```python
from build123d import *

# Parameters (mm, degrees)
SALIENTE_EXTRUIR1_DEPTH = 120
CROQUIS3_R              = 3.9
CORTAR_EXTRUIR1_DEPTH   = 32


with BuildPart() as part:
    # Croquis2 → Saliente-Extruir1 (new body)
    with BuildSketch(Plane(origin=(0, 0, 0), x_dir=(1, 0, 0), z_dir=(0, 1, 0))):
        with BuildLine():
            Line((-44.836996695, 15.45631068), (-20.836996695, 15.45631068))
            ThreePointArc((-20.836996695, 15.45631068), (-18.00856957, 14.284737804), (-16.836996695, 11.45631068))
            Line((-16.836996695, 11.45631068), (-16.836996695, -12.54368932))
            ThreePointArc((-16.836996695, -12.54368932), (-18.00856957, -15.372116445), (-20.836996695, -16.54368932))
            Line((-20.836996695, -16.54368932), (-44.836996695, -16.54368932))
            ThreePointArc((-44.836996695, -16.54368932), (-47.665423819, -15.372116445), (-48.836996695, -12.54368932))
            Line((-48.836996695, -12.54368932), (-48.836996695, 11.45631068))
            ThreePointArc((-48.836996695, 11.45631068), (-47.665423819, 14.284737804), (-44.836996695, 15.45631068))
        make_face()
    extrude(amount=SALIENTE_EXTRUIR1_DEPTH)

    # Croquis3 → Cortar-Extruir1 (cut)
    with BuildSketch(Plane.XY.offset(16.54368932)):
        with Locations((-32.836996695, 18)):
            Circle(CROQUIS3_R)
    extrude(amount=-CORTAR_EXTRUIR1_DEPTH, mode=Mode.SUBTRACT)


solid = part.part
```
The listing builds one solid part. Answer for the finished solid, in the listing's coordinates (mm). Give positions to 0.01 mm unless a question says otherwise; leave off trailing zeros. Order: outer loops, then holes, each group sorted by start corner. A loop starts at its lowest first (then second) coordinate and runs counter-clockwise, first axis right, second up.
1) Determine the mould class of faces 1 (the face through (-36.733, 18.171, 0.768)), 2 (the face through (-33, 0, 0)), 3 (the face through (-48.837, 59, 1)) for opening direction Y: pulls with the +Y half, pulls with the -Y half, needs draft (parallel to the pull), parting line crosses it, or undercut.
Reported:
face 1: undercut
face 2: pulls with the -Y half
face 3: needs draft
2) Consider line 1 along X through (y, z) = (49, -13); line 2 along X through (y, z) = (11, 14.5). Determine where each line is inside the solid, lowest interval first.
Reported:
line 1: x = -48.53 to -17.15
line 2: x = -48.33 to -17.35
3) Find section A-A on y = 18. Write down the section's boundary in (x, z), then the cut area to 3 significant figures.
Reported:
outline: (-48.84, -11.46) arc R4 ccw to (-44.84, -15.46) - (-36.74, -15.46) - (-36.74, 16.54) - (-44.84, 16.54) arc R4 ccw to (-48.84, 12.54) - close; (-28.94, -15.46) - (-20.84, -15.46) arc R4 ccw to (-16.84, -11.46) - (-16.84, 12.54) arc R4 ccw to (-20.84, 16.54) - (-28.94, 16.54) - close
area: 761 mm2
